Source: CAD feature listing. Evaluate the final solid. Frame: model axes, mm. A direction names the side the tool comes from. Give positions to 0.01 mm unless a question says otherwise; leave off trailing zeros. Loops run counter-clockwise (first coordinate to the right, second up) from the corner with the lowest first, then second, coordinate; pieces in that order, holes last. Notation, with made-up numbers: M -28,54 L 24,54 A19 cw 24,62 Z; hole C -38.5,4.25 d2. An arc over 180 degrees is marked long. Put each result on its own line as item: value.
from build123d import *

# Parameters (mm, degrees)
SKETCH1_W           = 130.81
SKETCH1_H           = 66.04
BOSS_EXTRUDE1_DEPTH = 36.83
FILLET1_R           = 2.54
SKETCH2_W           = 10.16
SKETCH2_H           = 15.24
BOSS_EXTRUDE2_DEPTH = 22.86
SKETCH3_W           = 13
SKETCH3_H           = 4.064
BOSS_EXTRUDE3_DEPTH = 9.525
SKETCH4_W           = 4.872
SKETCH4_H           = 5.08
CUT_EXTRUDE1_DEPTH  = 92.445213926


with BuildPart() as part:
    # Sketch1 → Boss-Extrude1 (new body)
    with BuildSketch(Plane(origin=(0, 0, 0), x_dir=(1, 0, 0), z_dir=(0, 1, 0))):
        Rectangle(SKETCH1_W, SKETCH1_H)
    extrude(amount=BOSS_EXTRUDE1_DEPTH)

    # Fillet1
    fillet1_edges = [part.edges().sort_by_distance(p)[0] for p in [
        (65.405, 36.83, 0),
        (0, 36.83, -33.02),
        (-65.405, 36.83, 0),
        (0, 0, -33.02),
        (65.405, 0, 0),
        (0, 0, 33.02),
        (-65.405, 0, 0),
        (0, 36.83, 33.02),
        (-65.405, 18.415, -33.02),
        (65.405, 18.415, -33.02),
        (65.405, 18.415, 33.02),
        (-65.405, 18.415, 33.02),
    ]]
    fillet(fillet1_edges, radius=FILLET1_R)

    # Sketch2 → Boss-Extrude2 (add)
    with BuildSketch(Plane(origin=(0, 36.83, 0), x_dir=(1, 0, 0), z_dir=(0, 1, 0))):
        with Locations((-19.685, 21.59)):
            Rectangle(SKETCH2_W, SKETCH2_H)
    extrude(amount=BOSS_EXTRUDE2_DEPTH)

    # Sketch3 → Boss-Extrude3 (add)
    with BuildSketch(Plane(origin=(0, 0, -33.02), x_dir=(-1, 0, 0), z_dir=(0, 0, -1))):
        with Locations((5.905, 9.968)):
            Rectangle(SKETCH3_W, SKETCH3_H)
    extrude(amount=BOSS_EXTRUDE3_DEPTH)

    # Sketch4 → Cut-Extrude1 (cut, through all)
    with BuildSketch(Plane(origin=(0, 12, 0), x_dir=(1, 0, 0), z_dir=(0, 1, 0))):
        with Locations((-5.905, 37.973)):
            Rectangle(SKETCH4_W, SKETCH4_H)
    extrude(amount=-CUT_EXTRUDE1_DEPTH, mode=Mode.SUBTRACT)


solid = part.part
1. Access query for faces 1 (the flat face through (-12.405, 10, -38)), 2 (the flat face through (-8.341, 10, -38)), 3 (the flat face through (-20, 48, -13.97)). Directions: +Z, -Z, +X, -X, +Y, -Y. A direction counts if a zero-diameter tool reaches every point of the face in a straight line with its end or side. Return the directions, or none.
Found:
face 1: -Z, -X, +Y, -Y
face 2: +Y, -Y
face 3: +Z, +X, -X, +Y
2. Contact query for flat-ended pins moving along their axis: P1, Ø8, axis at x = 4, z = 2, coming from the +Y side; P2, Ø7.5, axis at y = 50, z = -22, coming from the -X side (3 decimals); P3, Ø10.5, axis at x = -8, z = -36.5, coming from the -Y side; P4, Ø2, axis at y = 39.5, z = -31.5, coming from the +X side. Output: stop coordinate, or through.
Found:
P1: y = 36.83
P2: x = -24.765
P3: y = 0.12
P4: through
3. Material intervals for line 1 (Z direction, x = -19, y = 52.5); line 2 (Y direction, x = -32.5, z = -26); line 3 (Z direction, x = 13, y = 18), sorted ascending. Write a range as from..to.
Found:
line 1: -29.21..-13.97
line 2: 0..36.83
line 3: -33.02..33.02
4. Draft query along X for faces 4 (the flat face through (-9, 12, -38)), 5 (the cylindrical face through (-64.681, 18.637, -32.256)), 6 (the flat face through (-6, 10, -35.433)). Return one class per face: pulls with the +X half, pulls with the -X half, needs draft (parallel to the pull), parting line crosses it, or undercut.
Found:
face 4: needs draft
face 5: pulls with the -X half
face 6: undercut
5. Section query C-C (z = 24). Output: boundary loops of the cut face in (x, y) (3 decimals).
Found:
outline: M -65.405,2.54 A2.54 ccw -62.865,0 L 62.865,0 A2.54 ccw 65.405,2.54 L 65.405,34.29 A2.54 ccw 62.865,36.83 L -62.865,36.83 A2.54 ccw -65.405,34.29 Z
6. Section query A-A (x = -11). Output: boundary loops of the cut face in (y, z) (3 decimals).
Found:
outline: M 0,-30.48 A2.54 ccw 2.54,-33.02 L 7.936,-33.02 L 7.936,-42.545 L 12,-42.545 L 12,-33.02 L 34.29,-33.02 A2.54 ccw 36.83,-30.48 L 36.83,30.48 A2.54 ccw 34.29,33.02 L 2.54,33.02 A2.54 ccw 0,30.48 Z
7. Section query B-B (y = 22). Output: boundary loops of the cut face in (x, z) (3 decimals), plus the area to 3 significant figures.
Found:
outline: M -65.405,-30.48 A2.54 ccw -62.865,-33.02 L 62.865,-33.02 A2.54 ccw 65.405,-30.48 L 65.405,30.48 A2.54 ccw 62.865,33.02 L -62.865,33.02 A2.54 ccw -65.405,30.48 Z
area: 8,630 mm^2
8. Section query D-D (y = 56.5). Output: boundary loops of the cut face in (x, z) (3 decimals).
Found:
outline: M -24.765,-29.21 L -14.605,-29.21 L -14.605,-13.97 L -24.765,-13.97 Z
